The drawing under review shows one solid part. Ordinate dimensions are in mm from its lowest x, y, z. A direction names the side the tool comes from. Round coordinates to 2 decimals unless told otherwise and drop trailing zeros. Order: outer loops, then holes, each group sorted by start corner. A loop starts at its lowest first (then second) coordinate and runs counter-clockwise, first axis right, second up. Notation, with made-up numbers: (3.5, 88.25) -> (52.5, 88.25) arc R25 cw to (52.5, 113.25) -> close; hole circle Ø8 at (65.25, 82.5). An arc over 180 degrees is marked (long way). Use a Markdown table: item, result. Add a question column.
1) Consider section C-C (z = 1). State the section outline as (x, y) points (3 decimals).
2) Consider section B-B (x = 7.62). State the section outline as (y, z) points (1 decimal).
3) Wall thickness on line 1 along X through (y, z) = (0.65, 3) (3 decimals); line 2 along X through (y, z) = (0.3, 1) (3 decimals); line 3 along X through (y, z) = (0.85, 2.25) (3 decimals): over which ranges is each line inside the solid? List them lowest first. Write a range as [from, to].
4) Machinability: for the marked faces 1 and 2, which of the approach directions +Z, -Z, +X, -X, +Y, -Y give a long, thin tool a straight path to every point of the face, cutting with its end or side? Answer none if there is none.
5) Consider section A-A (y = 1.5). State the section outline as (x, z) points (1 decimal), plus the area to 3 significant figures.
6) Consider section D-D (x = 4). State the section outline as (y, z) points (3 decimals), plus the area to 3 significant figures.
7) Draft analysis for pull direction X (two halves, no side actions). For the marked faces 3, 4, 5 and 6, state which applies: pulls with the +X half, pulls with the -X half, needs draft (parallel to the pull), parting line crosses it, or undercut.
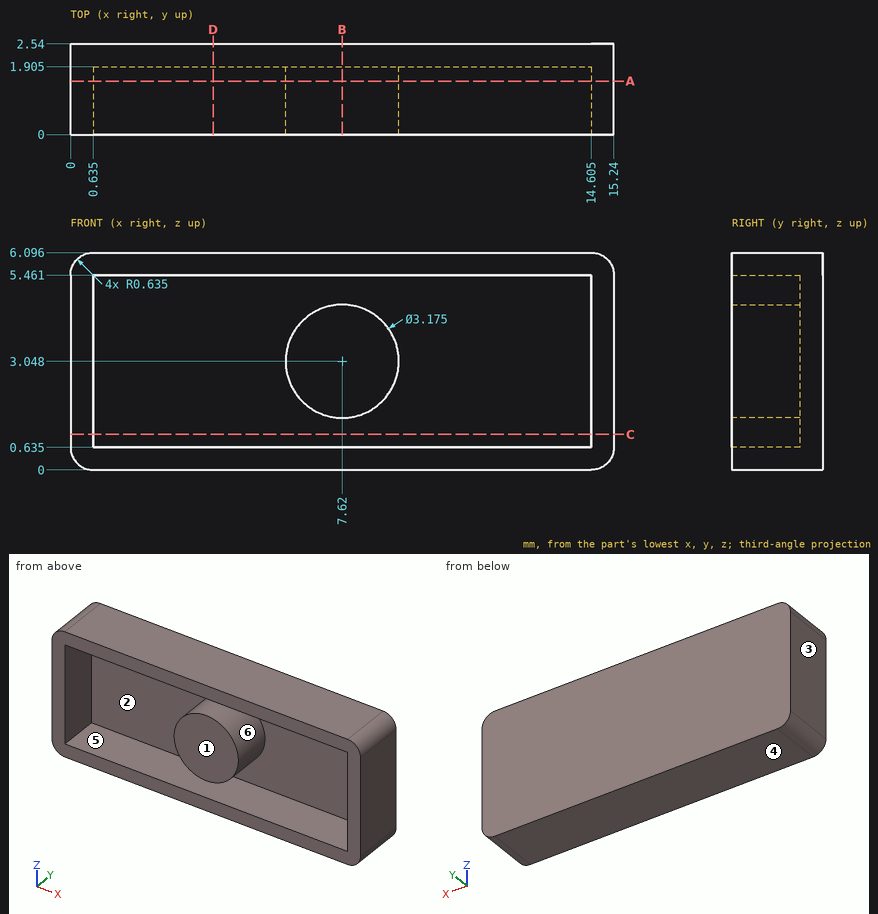
Results list:
| question | item | result |
|---|---|---|
| 1 | outline | (0, 0) -> (0.635, 0) -> (0.635, 1.905) -> (14.605, 1.905) -> (14.605, 0) -> (15.24, 0) -> (15.24, 2.54) -> (0, 2.54) -> close |
| 2 | outline | (0, 0) -> (2.5, 0) -> (2.5, 6.1) -> (0, 6.1) -> (0, 5.5) -> (1.9, 5.5) -> (1.9, 4.6) -> (0, 4.6) -> (0, 1.5) -> (1.9, 1.5) -> (1.9, 0.6) -> (0, 0.6) -> close |
| 3 | line 1 | [0, 0.635], [6.033, 9.207], [14.605, 15.24] |
| 3 | line 2 | [0, 0.635], [14.605, 15.24] |
| 3 | line 3 | [0, 0.635], [6.248, 8.992], [14.605, 15.24] |
| 4 | face 1 | +Z, -Z, +X, -X, -Y |
| 4 | face 2 | -Y |
| 5 | outline | (0, 0.6) arc R0.6 ccw to (0.6, 0) -> (14.6, 0) arc R0.6 ccw to (15.2, 0.6) -> (15.2, 5.5) arc R0.6 ccw to (14.6, 6.1) -> (0.6, 6.1) arc R0.6 ccw to (0, 5.5) -> close; circle Ø3.2 at (7.6, 3); hole (0.6, 0.6) -> (14.6, 0.6) -> (14.6, 5.5) -> (0.6, 5.5) -> close |
| 5 | area | 33.1 mm2 |
| 6 | outline | (0, 0) -> (2.54, 0) -> (2.54, 6.096) -> (0, 6.096) -> (0, 5.461) -> (1.905, 5.461) -> (1.905, 0.635) -> (0, 0.635) -> close |
| 6 | area | 6.29 mm2 |
| 7 | face 3 | pulls with the -X half |
| 7 | face 4 | needs draft |
| 7 | face 5 | undercut |
| 7 | face 6 | undercut |
